from build123d import *

# Parameters (mm, degrees)
F1_DEPTH = 30
F3_R     = 11.5
F4_DEPTH = 30
F2_R     = 11.5
F5_DEPTH = 90
F6_R     = 14.99999


# Not quite as in the source:
# - a fillet or chamfer is up to 0.001 mm smaller than in the source, because OpenCascade refuses the exact size


with BuildPart() as f1:
    # F0 (on Top) → F1 (new body)
    with BuildSketch(Plane.XY):
        Polygon((15, -15), (45, -15), (45, 15), (-45, 15), (-45, -15), (-15, -15), align=None)
        Polygon((15, -45), (15, -15), (-15, -15), (-15, -45), (0, -45), align=None)
    extrude(amount=F1_DEPTH)

    # F3 (on face) → F4 (cut)
    with BuildSketch(Plane.XZ.offset(45)):
        with Locations((0, 15)):
            Circle(F3_R)
    extrude(amount=-F4_DEPTH, mode=Mode.SUBTRACT)

    # F2 (on face) → F5 (cut)
    with BuildSketch(Plane(origin=(-45, 0, 0), x_dir=(0, -1, 0), z_dir=(-1, 0, 0))):
        with Locations((0, 15)):
            Circle(F2_R)
    extrude(amount=-F5_DEPTH, mode=Mode.SUBTRACT)

    # F6 (radius 15 in the source; OpenCascade refuses exactly that, so slightly less here)
    f6_edges = [f1.edges().sort_by_distance(p)[0] for p in [
        (0, 15, 0),
        (0, 15, 30),
    ]]
    fillet(f6_edges, radius=F6_R)


solid = f1.part
Verification items for the finished model (mm, model axes). A direction names the side the tool comes from. Coordinates: 2 decimals unless noted, no trailing zeros. Write each loop counter-clockwise with the first axis right and the second up, starting at its lowest first coordinate (ties: lowest second). Pieces come first, ordered by that corner, then holes. Notation, with made-up numbers: (-24.5, 83.25) - (6.5, 83.25) arc R34 cw to (6.5, 121.25) - close; hole circle Ø3 at (0, 84). An arc over 180 degrees is marked (long way). Answer as a JSON object with one key per item and string values.
(1) Cross-section at B-B on y = -33. Record the cut outline in (x, z), plus the area to 3 significant figures.
Report:
{"outline": "(-15, 0) - (15, 0) - (15, 30) - (-15, 30) - close; hole circle Ø23 at (0, 15)", "area": "485 mm^2"}
(2) Cross-section at C-C on z = 23. Record the cut outline in (x, y), plus the area to 3 significant figures.
Report:
{"outline": "(-45, -15) - (-15, -15) - (-15, -45) - (-8.26, -45) - (-8.26, -15) - (8.26, -15) - (8.26, -45) - (15, -45) - (15, -15) - (45, -15) - (45, -8.26) - (-45, -8.26) - close; (-45, 8.26) - (45, 8.26) - (45, 12.69) - (-45, 12.69) - close", "area": "1,410 mm^2"}
(3) Mould release check, pull along Z, two halves, no side actions. Record for faces 6 (the flat face through (15, -30, 15)), 7 (the cylindrical face through (-0.63, 10.49, 4.28)), 8 (the cylindrical face through (-0.6, 1.5, 26.4)): pulls with the +Z half, pulls with the -Z half, needs draft (parallel to the pull), parting line crosses it, or undercut.
Report:
{"face 6": "needs draft", "face 7": "pulls with the -Z half", "face 8": "undercut"}
(4) Tool access check on faces 1 (the flat face through (-45, -10, 21)), 2 (the flat face through (30, -15, 15)), 3 (the cylindrical face through (-0.63, 10.49, 25.72)), 4 (the cylindrical face through (-1.5, -30.2, 26.4)), 5 (the flat face through (-15, -30, 15)). Record the directions out of +Z, -Z, +X, -X, +Y, -Y that give a thin tool (end or side, any length) a straight path to the whole face; none if there is none.
Report:
{"face 1": "+Z, -Z, -X, +Y, -Y", "face 2": "+Z, -Z, +X, -Y", "face 3": "+Z, +X, -X, +Y", "face 4": "-Y", "face 5": "+Z, -Z, -X, -Y"}
(5) Thickness scan on line 1 along Z through (x, y) = (12, 0); line 2 along X through (y, z) = (-43, 14); line 3 along Y through (x, z) = (-4, 10). Record the ranges inside material, lowest first.
Report:
{"line 1": "0 to 3.5, 26.5 to 30", "line 2": "-15 to -11.46, 11.46 to 15", "line 3": "-15 to -10.36, 10.36 to 14.14"}
(6) Gauge pin test, flat ends, axial feed: pin 1 Ø4 at (y, z) = (-37, 21) entering from +X; pin 2 Ø2 at (x, z) = (-0.5, 10) entering from -Y; pin 3 Ø1 at (y, z) = (-19, 19.5) entering from -X. Record the tip position at first contact, or that the pin passes through.
Report:
{"pin 1": "x = 15", "pin 2": "y = -15", "pin 3": "x = -15"}
